Here's how the part is built. I have some questions about the finished solid (model axes, mm). A direction names the side the tool comes from. Coordinates: 2 decimals unless noted, no trailing zeros. Write each loop counter-clockwise with the first axis right and the second up, starting at its lowest first coordinate (ties: lowest second). Pieces come first, ordered by that corner, then holes. Notation, with made-up numbers: M 25,68 L 34,68 A14 cw 34,73 Z; hole C 58.5,30.25 d9. An arc over 180 degrees is marked long. Use a Markdown table: item, result.
Autodesk Inventor part; units mm, degrees
ref_plane "YZ Plane" through (0, 0, 0) normal (1, 0, 0) x (0, 1, 0)
ref_plane "XZ Plane" through (0, 0, 0) normal (0, 1, 0) x (-1, 0, 0)
ref_plane "XY Plane" through (0, 0, 0) normal (0, 0, 1) x (1, 0, 0)
sketch "Sketch1" plane through (0, 0, 0) normal (0, 0, 1) x (1, 0, 0)
  line L0 (-13, -1.75) -> (13, -1.75)
  line L1 (13, -1.75) -> (13, 1.75)
  line L2 (13, 1.75) -> (-13, 1.75)
  line L3 (-13, 1.75) -> (-13, -1.75)
  line L4 (-13, -1.75) -> (13, 1.75) construction
  line L5 (13, -1.75) -> (-13, 1.75) construction
  line L6 (0, 1.75) -> (0, 5.75)
  circle A0 centre (0, 5.75) radius 4
  circle A1 centre (0, 5.75) radius 5.75
  line L7 (-5.75, 5.75) -> (-5.75, 1.75)
  line L8 (5.75, 5.75) -> (5.75, 1.75)
  point P0 (0, 0)
  dimension "d0" = 26
  dimension "d1" = 3.5
  dimension "d2" = 4
  dimension "d3" = 8
  dimension "d4" = 11.5
extrude "Extrusion1" add sketch "Sketch1" along normal blind 7.25
sketch "Sketch2" plane through (-13, -1.75, 0) normal (0, -1, 0) x (1, 0, 0)
  line L0 (13, 0) -> (13, 7.25)
  line L1 (9, 7.25) -> (17, 7.25)
  line L2 (13, 3.625) -> (22.375, 3.625)
  line L3 (22.375, 3.625) -> (3.625, 3.625)
  circle A0 centre (22.375, 3.625) radius 1.6
  circle A1 centre (3.625, 3.625) radius 1.6
  dimension "d7" = 9.375
  dimension "d8" = 18.75
  dimension "d9" = 3.2
  dimension "d10" = 3.2
extrude "Extrusion2" cut sketch "Sketch2" against normal blind 7.25
properties part number "Mauch_Power_Button_Bracket" material "ABS Plastic"
1. Suppose I cut it at B-B on z = 5.5. Write out the boundary of the cut face in (x, y), and give its area (3 significant figures).
Answers follow:
| item | result |
|---|---|
| outline | M -13,-1.75 L 13,-1.75 L 13,1.75 L 5.75,1.75 L 5.75,5.75 A5.75 ccw -5.75,5.75 L -5.75,1.75 L -13,1.75 Z; hole C 0,5.75 d8 |
| area | 139 mm2 |
2. We'd pull the mould along Z, two halves only. Please class faces 4 (the face through (-7.7, 1.75, 2.8)), 5 (the face through (-10.973, -0.024, 3.695)), 6 (the face through (0, 1, 7.25)): +Z half, -Z half, draft (parallel to the pull), parting line (faces both ways), or undercut.
Answers follow:
| item | result |
|---|---|
| face 4 | draft |
| face 5 | undercut |
| face 6 | +Z half |
3. Which directions (+Z, -Z, +X, -X, +Y, -Y) give clear straight access to the entire face, cutting with the end or side of a thin tool? Please do faces 1 (the face through (-5.75, 4, 4)), 2 (the face through (-0.1, 11.5, 3.6)), 3 (the face through (5.75, 4, 4)).
Answers follow:
| item | result |
|---|---|
| face 1 | +Z, -Z, -X, +Y |
| face 2 | +Z, -Z, +Y |
| face 3 | +Z, -Z, +X, +Y |
4. Suppose I cut it at D-D on y = 1.5. Write out the boundary of the cut face in (x, z) (3 decimals), and give its area (3 significant figures).
Answers follow:
| item | result |
|---|---|
| outline | M -13,0 L 13,0 L 13,7.25 L -13,7.25 Z; hole C -9.375,3.625 d3.2; hole C 9.375,3.625 d3.2 |
| area | 172 mm2 |
5. I need wall thicknesses on probe 1 along X at (y, z) = (5.75, 2.75); probe 2 along Y at (x, z) = (0, 3); probe 3 along Y at (x, z) = (1.5, 1.25). Which ranges of each line are inside material? Lowest first, please.
Answers follow:
| item | result |
|---|---|
| probe 1 | x = -5.75 to -4, 4 to 5.75 |
| probe 2 | y = -1.75 to 1.75, 9.75 to 11.5 |
| probe 3 | y = -1.75 to 2.04, 9.46 to 11.3 |
6. Suppose I cut it at C-C on y = 8.25. Write out the boundary of the cut face in (x, z).
Answers follow:
| item | result |
|---|---|
| outline | M -5.18,0 L -3.12,0 L -3.12,7.25 L -5.18,7.25 Z; M 3.12,0 L 5.18,0 L 5.18,7.25 L 3.12,7.25 Z |
7. Will these pins go through, and if not, where does the flat tip stop? pin 1 Ø1 at (y, z) = (7, 1.5) entering from -X; pin 2 Ø1.2 at (y, z) = (4, 4.5) entering from -X; pin 3 Ø2 at (y, z) = (4, 4) entering from +X; pin 4 Ø5 at (x, y) = (0, 5.75) entering from -Z.
Answers follow:
| item | result |
|---|---|
| pin 1 | stops at x = -5.7 |
| pin 2 | stops at x = -5.75 |
| pin 3 | stops at x = 5.75 |
| pin 4 | passes through |
8. Suppose I cut it at A-A on x = 0. Write out the boundary of the cut face in (y, z).
Answers follow:
| item | result |
|---|---|
| outline | M -1.75,0 L 1.75,0 L 1.75,7.25 L -1.75,7.25 Z; M 9.75,0 L 11.5,0 L 11.5,7.25 L 9.75,7.25 Z |
